Here's the drawing with two shaded views (mm, measured from the low corner). I have some questions. A direction names the side the tool comes from. Round coordinates to 2 decimals unless told otherwise and drop trailing zeros. Loops run counter-clockwise (first coordinate to the right, second up) from the corner with the lowest first, then second, coordinate; pieces in that order, holes last.
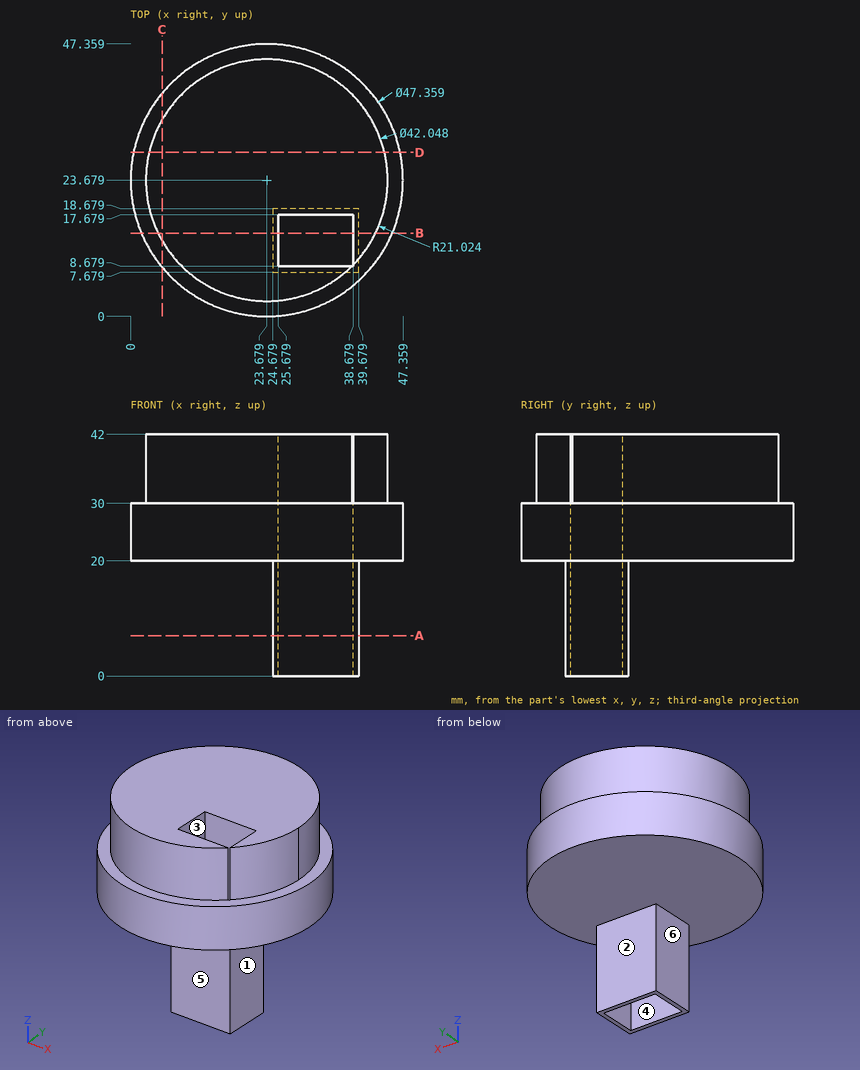
(1) If we section it at B-B, the plane y = 14.5: List the corners of the cut face in (x, z) for me (1 decimal).
Worked answers:
outline: (1.9, 20) - (24.7, 20) - (24.7, 0) - (25.7, 0) - (25.7, 42) - (4.8, 42) - (4.8, 30) - (1.9, 30) - close; (38.7, 0) - (39.7, 0) - (39.7, 20) - (45.5, 20) - (45.5, 30) - (42.6, 30) - (42.6, 42) - (38.7, 42) - close
(2) If we section it at C-C, the plane x = 5.5: List the corners of the cut face in (y, z) for me, then the cut area to 3 significant figures.
Worked answers:
outline: (8.51, 20) - (38.85, 20) - (38.85, 30) - (34.24, 30) - (34.24, 42) - (13.12, 42) - (13.12, 30) - (8.51, 30) - close
area: 557 mm2
(3) If we mould it in two halves opening along X, with no side actions, what happens to the marked faces 4, 5 and 6? For each: released by +X, released by -X, zero draft, split by the parting line, or undercut.
Worked answers:
face 4: undercut
face 5: zero draft
face 6: released by -X
(4) If we section it at A-A, the plane z = 7: List the corners of the cut face in (x, y) for me.
Worked answers:
outline: (24.68, 7.68) - (39.68, 7.68) - (39.68, 18.68) - (24.68, 18.68) - close; hole (25.68, 8.68) - (38.68, 8.68) - (38.68, 17.68) - (25.68, 17.68) - close
(5) If we section it at D-D, the plane y = 28.5: List the corners of the cut face in (x, z) for me (1 decimal).
Worked answers:
outline: (0.5, 20) - (46.9, 20) - (46.9, 30) - (44.1, 30) - (44.1, 42) - (3.2, 42) - (3.2, 30) - (0.5, 30) - close
(6) Will these pins go through, and if not, where does the flat tip stop? P1, Ø5, axis at x = 16.5, z = 21, coming from the -Y side; P2, Ø10.5, axis at x = 29.5, z = 21, coming from the -Y side; P3, Ø10, axis at x = 8.5, z = 25, coming from the +Y side.
Worked answers:
P1: stops at y = 0.47
P2: stops at y = 0.01
P3: stops at y = 45.06
(7) For the marked faces 1, 2 and 3, which set-ups out of +Z, -Z, +X, -X, +Y, -Y let a thin tool reach every point of the face, with its end or its side?
Worked answers:
face 1: -Z, +X, +Y, -Y
face 2: -Z, +X, -X, +Y
face 3: +Z, -Z
(8) If I drill on line 1 (X direction, y = 12, z = 12); line 2 (Y direction, x = 27, z = 11.5); line 3 (Z direction, x = 37.5, y = 24.5), over which ranges is the centre line in solid material (lowest first)?
Worked answers:
line 1: x = 24.68 to 25.68, 38.68 to 39.68
line 2: y = 7.68 to 8.68, 17.68 to 18.68
line 3: z = 20 to 42
